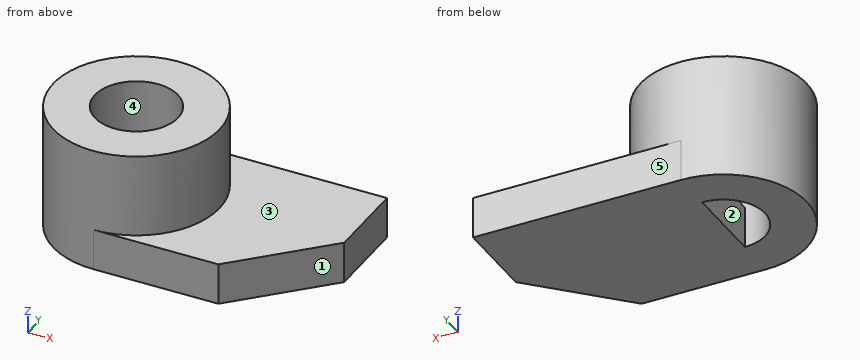
from build123d import *

# Parameters (mm, degrees)
F0_R     = 12.7
F0_R_2   = 6.35
F1_DEPTH = 19.05
F2_W     = 31.75
F2_H     = 6.35
F3_DEPTH = 12.7
F5_DEPTH = 6.35


with BuildPart() as f1:
    # F0 (on Top) → F1 (new body)
    with BuildSketch(Plane.XY):
        Circle(F0_R)
        Circle(F0_R_2, mode=Mode.SUBTRACT)
    extrude(amount=F1_DEPTH)

    # F2 (on Front) → F3 (join, symmetric)
    with BuildSketch(Plane.XZ):
        with Locations((15.875, 3.175)):
            Rectangle(F2_W, F2_H)
    extrude(amount=F3_DEPTH, both=True)

    # F4 (on face) → F5 (cut)
    with BuildSketch(Plane.XY.offset(6.35)):
        Polygon((31.75, -12.7), (31.75, 0), (19.05, -12.7), align=None)
    extrude(amount=-F5_DEPTH, mode=Mode.SUBTRACT)


solid = f1.part
Can you work these out from the model? Positions are in its coordinate system, mm. Face numbers are marked on the shaded views. A direction names the side the tool comes from. Round coordinates to 2 decimals unless told otherwise and drop trailing zeros. Loops run counter-clockwise (first coordinate to the right, second up) from the corner with the lowest first, then second, coordinate; pieces in that order, holes last. Notation, with made-up numbers: (27.5, 74) - (71.5, 74) arc R13 cw to (71.5, 82) - close; hole circle Ø11 at (41, 41). An arc over 180 degrees is marked (long way). Write item = value, one per line. Start each with the question number.
(1) For the marked faces 4 and 5, which set-ups out of +Z, -Z, +X, -X, +Y, -Y let a thin tool reach every point of the face, with its end or its side?
(2) If we section it at B-B (z = 11.5): Please give me the cut outline in (x, y).
(3) If we section it at A-A (x = -2.5): Please give me the cut outline in (y, z).
(4) If we section it at D-D (x = 11): Please give me the cut outline in (y, z).
(5) If we section it at C-C (y = -0.5): Please give me the cut outline in (x, z), and give its area (3 significant figures).
(6) If I drill on probe 1 along X at (y, z) = (0, 5.25); probe 2 along Y at (x, z) = (0, 11), over which ranges is the centre line in solid material (lowest first)? Write a range as [from, to].
(7) If we mould it in two halves opening along X, with no side actions, what happens to the marked faces 1, 2 and 3? For each: released by +X, released by -X, zero draft, split by the parting line, or undercut.
(8) For P1, Ø1, axis at x = 9.5, z = 8, coming from the +Y side; P2, Ø3, axis at x = 10, z = 15, coming from the +Y side; P3, Ø3, axis at x = 22, y = 9, coming from the +Z side, each with a flat end and sliding along its axis, tell me the tip position at first contact or that it passes through.
Ans:
q1.face_4 = +Z
q1.face_5 = +Z, -Z, +X, -X, +Y
q2.outline = circle Ø25.4 at (0, 0); hole circle Ø12.7 at (0, 0)
q3.outline = (-12.45, 0) - (-5.84, 0) - (-5.84, 19.05) - (-12.45, 19.05) - close; (5.84, 0) - (12.45, 0) - (12.45, 19.05) - (5.84, 19.05) - close
q4.outline = (-12.7, 0) - (12.7, 0) - (12.7, 6.35) - (6.35, 6.35) - (6.35, 19.05) - (-6.35, 19.05) - (-6.35, 6.35) - (-12.7, 6.35) - close
q5.outline = (-12.69, 0) - (-6.33, 0) - (-6.33, 19.05) - (-12.69, 19.05) - close; (0, 0) - (31.25, 0) - (31.25, 6.35) - (12.69, 6.35) - (12.69, 19.05) - (6.33, 19.05) - (6.33, 6.35) - (0, 6.35) - close
q5.area = 400 mm²
q6.probe_1 = [-12.7, -6.35], [0, 31.75]
q6.probe_2 = [-12.7, -6.35], [6.35, 12.7]
q7.face_1 = released by +X
q7.face_2 = undercut
q7.face_3 = zero draft
q8.P1 = 8.96
q8.P2 = 9.44
q8.P3 = 6.35
